Build history of the part. All positions in model axes, mm. A direction names the side the tool comes from. Round coordinates to 2 decimals unless told otherwise and drop trailing zeros. Write each loop counter-clockwise with the first axis right and the second up, starting at its lowest first coordinate (ties: lowest second). Pieces come first, ordered by that corner, then holes.
Item 1: Band-saw the part on A-A, the plane x = 2. Write the cut outline in (y, z).
Item 2: Drop flat-ended pins along their axis: pin 1 Ø1.2 at (x, z) = (3, -26) entering from +Y; pin 2 Ø1.3 at (x, z) = (0.5, -13.5) entering from +Y; pin 3 Ø2 at (x, z) = (7.5, -20) entering from -Y; pin 4 Ø0.6 at (y, z) = (1.5, -27.5) entering from -X. Give the stop position or say it passes through.
Item 3: 3-axis set-ups, long thin cutter, end or side, ignore diameter. For faces 4 (the flat face through (6, 1, -23.2)), 5 (the flat face through (12, 1, -27)), 6 (the flat face through (1.2, 1, -7)), 7 (the flat face through (12, 2, -19)), 8 (the flat face through (17, 0.8, -17)): which of +Z, -Z, +X, -X, +Y, -Y reach the whole face in a straight line?
Item 4: Wall check: probe 1 along X at (y, z) = (1.05, -26.5); probe 2 along X at (y, z) = (0.55, -21); probe 3 along X at (y, z) = (0.75, -27.5). Give the ranges that are in metal, low to high.
Item 5: Band-saw the part on D-D, the plane z = -10. Write the cut outline in (x, y).
Item 6: Mould opens along X. For faces 1 (the flat face through (16, 1, -27)), 2 (the flat face through (11, 0, -17)), 3 (the flat face through (17.4, 0.4, -17)) say: +X half, -X half, draft (parallel to the pull), parting line (faces both ways), or undercut.
Item 7: Band-saw the part on B-B, the plane y = 1.2. Write the cut outline in (x, z).
Item 8: Band-saw the part on C-C, the plane z = -21.5. Write the cut outline in (x, y).
```python
from build123d import *

# Parameters (mm, degrees)
SKICA1_W                 = 17.4
SKICA1_H                 = 27
P_IDAT_VYSUNUT_M1_DEPTH  = 2
SKICA2_W                 = 17.4
SKICA2_H                 = 27
P_IDAT_VYSUNUT_M2_DEPTH  = 6
ZAOBLIT1_R               = 4
SKICA3_W                 = 17.4
SKICA3_H                 = 27
ODEBRAT_VYSUNUT_M1_DEPTH = 6
SKICA4_W                 = 1.2
SKICA4_H                 = 26.464101615
ODEBRAT_VYSUNUT_M2_DEPTH = 1.2
SKICA7_W                 = 15
SKICA7_H                 = 1.2
SKICA7_W_2               = 17.4
SKICA7_H_2               = 0.8
P_IDAT_VYSUNUT_M3_DEPTH  = 7
SKICA8_W                 = 9.2
SKICA8_H                 = 9.2
ODEBRAT_VYSUNUT_M5_DEPTH = 7
SKICA10_W                = 4
SKICA10_H                = 4
ODEBRAT_VYSUNUT_M6_DEPTH = 1.6


with BuildPart() as part:
    # Skica1 → Přidat vysunutím1 (new body)
    with BuildSketch(Plane(origin=(0, 0, 0), x_dir=(1, 0, 0), z_dir=(0, 1, 0))):
        with Locations((8.7, 13.5)):
            Rectangle(SKICA1_W, SKICA1_H)
    extrude(amount=P_IDAT_VYSUNUT_M1_DEPTH)

    # Skica2 → Přidat vysunutím2 (add)
    with BuildSketch(Plane.XZ):
        with Locations((8.7, -13.5)):
            Rectangle(SKICA2_W, SKICA2_H)
    extrude(amount=P_IDAT_VYSUNUT_M2_DEPTH)

    # Zaoblit1
    zaoblit1_edges = [part.edges().sort_by_distance(p)[0] for p in [
        (8.7, 2, 0),
    ]]
    fillet(zaoblit1_edges, radius=ZAOBLIT1_R)

    # Skica3 → Odebrat vysunutím1 (cut)
    with BuildSketch(Plane.XZ.offset(6)):
        with Locations((8.7, -13.5)):
            Rectangle(SKICA3_W, SKICA3_H)
    extrude(amount=-ODEBRAT_VYSUNUT_M1_DEPTH, mode=Mode.SUBTRACT)

    # Skica4 → Odebrat vysunutím2 (cut)
    with BuildSketch(Plane(origin=(0, 2, 0), x_dir=(1, 0, 0), z_dir=(0, 1, 0))):
        with Locations((0.6, 13.767949192)):
            Rectangle(SKICA4_W, SKICA4_H)
        with Locations((16.8, 13.767949192)):
            Rectangle(SKICA4_W, SKICA4_H)
    extrude(amount=-ODEBRAT_VYSUNUT_M2_DEPTH, mode=Mode.SUBTRACT)

    # Skica7 → Přidat vysunutím3 (add)
    with BuildSketch(Plane(origin=(0, 0, -27), x_dir=(-1, 0, 0), z_dir=(0, 0, -1))):
        with Locations((-8.7, 1.4)):
            Rectangle(SKICA7_W, SKICA7_H)
        with Locations((-8.7, 0.4)):
            Rectangle(SKICA7_W_2, SKICA7_H_2)
    extrude(amount=P_IDAT_VYSUNUT_M3_DEPTH)

    # Skica8 → Odebrat vysunutím5 (cut)
    with BuildSketch(Plane(origin=(0, 2, 0), x_dir=(1, 0, 0), z_dir=(0, 1, 0))):
        with Locations((5.8, 18.6)):
            Rectangle(SKICA8_W, SKICA8_H)
    extrude(amount=-ODEBRAT_VYSUNUT_M5_DEPTH, mode=Mode.SUBTRACT)

    # Skica10 → Odebrat vysunutím6 (cut)
    with BuildSketch(Plane(origin=(0, 2, 0), x_dir=(1, 0, 0), z_dir=(0, 1, 0))):
        with Locations((3.4, 26.7)):
            Rectangle(SKICA10_W, SKICA10_H)
        with Locations((14, 26.7)):
            Rectangle(SKICA10_W, SKICA10_H)
    extrude(amount=-ODEBRAT_VYSUNUT_M6_DEPTH, mode=Mode.SUBTRACT)


solid = part.part
```
Results:
1. outline: (0, -34) - (2, -34) - (2, -28.7) - (0.4, -28.7) - (0.4, -24.7) - (2, -24.7) - (2, -23.2) - (0, -23.2) - close; (0, -14) - (2, -14) - (2, -4) arc R4 ccw to (0, -0.54) - close
2. pin 1: stops at y = 0.4
2. pin 2: stops at y = 0.8
2. pin 3: passes through
2. pin 4: stops at x = 1.2
3. face 4: +Y, -Y
3. face 5: +Y
3. face 6: +Z, -Z, -X, +Y
3. face 7: +Z, -Z, +X, -X, +Y
3. face 8: +Z, -Z, +X, +Y
4. probe 1: x = 1.2 to 1.4, 5.4 to 12, 16 to 16.2
4. probe 2: x = 0 to 1.2, 10.4 to 17.4
4. probe 3: x = 0 to 1.4, 5.4 to 12, 16 to 17.4
5. outline: (0, 0) - (17.4, 0) - (17.4, 0.8) - (16.2, 0.8) - (16.2, 2) - (1.2, 2) - (1.2, 0.8) - (0, 0.8) - close
6. face 1: undercut
6. face 2: draft
6. face 3: +X half
7. outline: (1.2, -34) - (16.2, -34) - (16.2, -1.6) - (1.2, -1.6) - (1.2, -14) - (10.4, -14) - (10.4, -23.2) - (1.2, -23.2) - close; hole (1.4, -28.7) - (5.4, -28.7) - (5.4, -24.7) - (1.4, -24.7) - close; hole (12, -28.7) - (16, -28.7) - (16, -24.7) - (12, -24.7) - close
8. outline: (0, 0) - (1.2, 0) - (1.2, 0.8) - (0, 0.8) - close; (10.4, 0) - (17.4, 0) - (17.4, 0.8) - (16.2, 0.8) - (16.2, 2) - (10.4, 2) - close
